```python
from build123d import *

# Parameters (mm, degrees)
F1_DEPTH = 100
F2_W     = 20
F2_H     = 89.4427191
F3_DEPTH = 10
F4_DEPTH = 10


with BuildPart() as f1:
    # F0 (on Front) → F1 (new body)
    with BuildSketch(Plane.XZ):
        Polygon((20, 0), (0, 0), (0, -100), (100, -100), (100, -80), (60, 0), (40, 0), (40, -20), (20, -20), align=None)
    extrude(amount=F1_DEPTH)

    # F2 (on face) → F3 (cut)
    with BuildSketch(Plane(origin=(48, 0, 24), x_dir=(0, 1, 0), z_dir=(0.894427191, 0, 0.4472135955))):
        with Locations((-50, -71.55417528)):
            Rectangle(F2_W, F2_H)
    extrude(amount=-F3_DEPTH, mode=Mode.SUBTRACT)

    # F4 (cut): a face of the model
    f4_faces = [f1.faces().sort_by_distance(p)[0] for p in [
        (55.527864045, -50, -2.2360679775),
    ]]
    extrude(f4_faces, amount=-F4_DEPTH, mode=Mode.SUBTRACT)


solid = f1.part
```
Geometry check sheet. Reference: the model listing, model coordinates, mm. A direction names the side the tool comes from. Give positions to 0.01 mm unless a question says otherwise; leave off trailing zeros. Loops run counter-clockwise (first coordinate to the right, second up) from the corner with the lowest first, then second, coordinate; pieces in that order, holes last. Notation, with made-up numbers: M 9.25,37.5 L 27.25,37.5 A27 ccw 27.25,62.5 Z; hole C 59,-2.5 d10. An arc over 180 degrees is marked long. Write item = value, one per line.
(1) Sectioned sample at A-A, the plane y = -57.5. Record the cut outline in (x, z).
Answer below:
outline = M 0,-100 L 100,-100 L 100,-80 L 91.06,-84.47 L 48.82,0 L 40,0 L 40,-20 L 20,-20 L 20,0 L 0,0 Z
(2) Sectioned sample at D-D, the plane x = 57.5. Record the cut outline in (y, z), plus the area to 3 significant figures.
Answer below:
outline = M -100,-100 L 0,-100 L 0,0 L -40,0 L -40,-17.36 L -60,-17.36 L -60,0 L -100,0 Z
area = 9,650 mm2
(3) Gauge pin test, flat ends, axial feed: pin 1 Ø1.5 at (y, z) = (-21.5, -32.5) entering from +X (3 decimals); pin 2 Ø1 at (y, z) = (-42.5, -74.5) entering from +X; pin 3 Ø16 at (y, z) = (-61, -9.5) entering from +X. Record the tip position at first contact, or that the pin passes through.
Answer below:
pin_1 = 76.625
pin_2 = 86.32
pin_3 = 68.75
(4) Sectioned sample at C-C, the plane z = -33. Record the cut outline in (x, y), plus the area to 3 significant figures.
Answer below:
outline = M 0,-100 L 76.5,-100 L 76.5,-60 L 65.32,-60 L 65.32,-40 L 76.5,-40 L 76.5,0 L 0,0 Z
area = 7,430 mm2
(5) Tool access check on faces 1 (the face through (30, -49, -20)), 2 (the face through (49, -49, -100)), 3 (the face through (96, -50, -82)). Record the directions out of +Z, -Z, +X, -X, +Y, -Y that give a thin tool (end or side, any length) a straight path to the whole face; none if there is none.
Answer below:
face_1 = +Z, +Y, -Y
face_2 = -Z, +X, -X, +Y, -Y
face_3 = +Z
(6) Material ranges on line 1 (Y direction, x = 85, z = -52.5); line 2 (Z direction, x = 32.5, y = -73); line 3 (X direction, y = -37.5, z = -6.5), recorded low to high. Write a range as [from, to].
Answer below:
line_1 = [-100, -60], [-40, 0]
line_2 = [-100, -20]
line_3 = [0, 20], [40, 63.25]
(7) Sectioned sample at B-B, the plane z = -10.5. Record the cut outline in (x, y).
Answer below:
outline = M 0,-100 L 20,-100 L 20,0 L 0,0 Z; M 40,-100 L 65.25,-100 L 65.25,-60 L 54.07,-60 L 54.07,-40 L 65.25,-40 L 65.25,0 L 40,0 Z
(8) Release check for a two-part mould opening along X. For faces 4 (the face through (80.3, -79.7, -40.6)), 5 (the face through (40, -49, -10)), 6 (the face through (0, -49, -49)) record: released by +X, released by -X, zero draft, split by the parting line, or undercut.
Answer below:
face_4 = released by +X
face_5 = undercut
face_6 = released by -X
